CAD build for the part. Positions are in the model's coordinates, mm. Give positions to 0.01 mm unless a question says otherwise; leave off trailing zeros. Write each loop counter-clockwise with the first axis right and the second up, starting at its lowest first coordinate (ties: lowest second). Pieces come first, ordered by that corner, then holes. Notation, with made-up numbers: (69.25, 19) -> (75.25, 19) arc R32 ccw to (75.25, 50) -> close; hole circle Ø4 at (-3.75, 39.25). An arc over 180 degrees is marked (long way). Use one line per item in the form item = value. Start each with the question number.
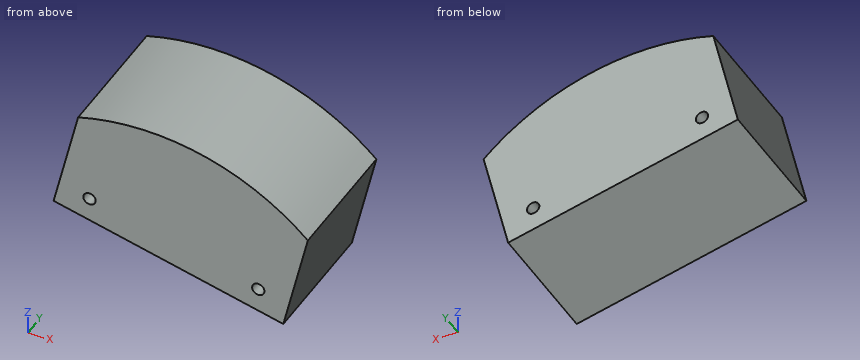
from build123d import *

# Parameters (mm, degrees)
BOSS_EXTRUDE1_DEPTH         = 50.8
F_12_0_189_DIAMETER_HOLE1_D = 4.8006


with BuildPart() as part:
    # Sketch1 → Boss-Extrude1 (new body)
    with BuildSketch(Plane(origin=(0, 0, 0), x_dir=(1, 0, 0), z_dir=(0, 1, 0))):
        with BuildLine():
            Line((63.017839503, -66.782093), (53.468205472, -26.506342671))
            Line((53.468205472, -26.506342671), (-35.875703335, -47.690346072))
            Line((-35.875703335, -47.690346072), (-26.326069304, -87.966096401))
            ThreePointArc((-26.326069304, -87.966096401), (21.184003401, -89.343908807), (63.017839503, -66.782093))
        make_face()
    extrude(amount=BOSS_EXTRUDE1_DEPTH)

    # #12 (0.189) Diameter Hole1 (through all)
    with Locations(Plane(origin=(0, 50.8, 0), x_dir=(1, 0, 0), z_dir=(0, 1, 0))):
        with Locations((-21.91216983, -53.736183096), (43.742627992, -38.169017556)):
            Hole(F_12_0_189_DIAMETER_HOLE1_D / 2)


solid = part.part
1) Cut at C-C (z = 84). Give the cut face in (x, y).
2) Cut at B-B (y = 25). Give the cut face in (x, z).
3) Wall check: line 1 along Z through (x, y) = (-23.5, 13); line 2 along Z through (x, y) = (-23, 17.5); line 3 along Z through (x, y) = (30.5, 23.5). Give the ranges that are in metal, low to high. Write a range as from..to.
4) Cut at A-A (x = -23). Give the cut face in (y, z), and give its area (3 significant figures).
5) Cut at D-D (x = 12.5). Give the cut face in (y, z).
6) Pin check, flat tips, straight feed: pin 1 (2 mm diameter, centred on x = 29, y = 16.5, fed in from +Z); pin 2 (12 mm diameter, centred on y = 34.5, z = 80, fed in from -X); pin 3 (5 mm diameter, centred on x = 21.5, y = 41.5, fed in from +Z). Stop position of each tip, or through.
Final values:
q1.outline = (-27.27, 0) -> (37.08, 0) -> (37.08, 50.8) -> (-27.27, 50.8) -> close
q2.outline = (-35.88, 47.69) -> (53.47, 26.51) -> (63.02, 66.78) arc R91.82 ccw to (-26.33, 87.97) -> close; hole circle Ø4.8 at (-21.91, 53.74); hole circle Ø4.8 at (43.74, 38.17)
q3.line_1 = 44.76..51.94, 55.54..88.76
q3.line_2 = 44.64..51.6, 55.88..88.89
q3.line_3 = 31.95..86.61
q4.outline = (0, 44.64) -> (50.8, 44.64) -> (50.8, 51.6) -> (0, 51.6) -> close; (0, 55.88) -> (50.8, 55.88) -> (50.8, 88.89) -> (0, 88.89) -> close
q4.area = 2,030 mm^2
q5.outline = (0, 36.22) -> (50.8, 36.22) -> (50.8, 90.97) -> (0, 90.97) -> close
q6.pin_1 = 87.45
q6.pin_2 = -29.64
q6.pin_3 = 89.83
